from build123d import *

# Parameters (mm, degrees)
SKETCH3_R               = 25.75
SKETCH3_R_2             = 23.75
BOSS_EXTRUDE1_DEPTH     = 82
SKETCH2_R               = 24.35
SKETCH2_R_2             = 22.35
BOSS_EXTRUDE2_DEPTH     = 30
CUT_EXTRUDE1_DEPTH      = 30
CUT_EXTRUDE1_DEPTH_BACK = 30
SKETCH5_W               = 101.816386604
SKETCH5_H               = 90.816460778
CUT_EXTRUDE2_DEPTH      = 30
SKETCH6_W               = 2
SKETCH6_H               = 20.775230247
BOSS_EXTRUDE3_DEPTH     = 61
BOSS_EXTRUDE5_DEPTH     = 25


with BuildPart() as part:
    # Sketch3 → Boss-Extrude1 (new body)
    with BuildSketch(Plane(origin=(-103.870896529, 742.017814767, 0), x_dir=(-0.9903438719336157, -0.13863266326351154, 0), z_dir=(0.13863266326351156, -0.9903438719336158, 0))):
        with Locations(Location((-535.354479902, 0, 0), (0, 0, 180))):
            Circle(SKETCH3_R)
        with Locations(Location((-535.354479902, 0, 0), (0, 0, 180))):
            Circle(SKETCH3_R_2, mode=Mode.SUBTRACT)
    extrude(amount=-BOSS_EXTRUDE1_DEPTH)

    # Sketch4 → Cut-Extrude1 (cut, two sides: drawn at the far end of the back side and taken through both)
    with BuildSketch(Plane.XY.offset(-CUT_EXTRUDE1_DEPTH_BACK)):
        Polygon((414.924769966, 897.597101018), (426.314131953, 816.235432106), (451.815486656, 819.805223185), (440.426124669, 901.166892097), align=None)
    extrude(amount=CUT_EXTRUDE1_DEPTH + CUT_EXTRUDE1_DEPTH_BACK, mode=Mode.SUBTRACT)


with BuildPart() as body_2:
    # Sketch2 → Boss-Extrude2 (new body)
    with BuildSketch(Plane(origin=(455.481917253, 0, 0), x_dir=(0, 0, -1), z_dir=(1, 0, 0))):
        with Locations((0, 857.898759871)):
            Circle(SKETCH2_R)
        with Locations((0, 857.898759871)):
            Circle(SKETCH2_R_2, mode=Mode.SUBTRACT)
    extrude(amount=BOSS_EXTRUDE2_DEPTH)


with BuildPart() as cut_extrude2_tool:
    # Sketch5 → Cut-Extrude2 (new body)
    with BuildSketch(Plane.XY):
        with Locations((437.415428166, 854.729783017)):
            Rectangle(SKETCH5_W, SKETCH5_H)
    extrude(amount=-CUT_EXTRUDE2_DEPTH)


with BuildPart() as part_1:
    add(part.part)

    # Cut-Extrude2: cut by cut_extrude2_tool
    add(cut_extrude2_tool.part, mode=Mode.SUBTRACT)



with BuildPart() as body_2_1:
    add(body_2.part)

    # Cut-Extrude2: cut by cut_extrude2_tool
    add(cut_extrude2_tool.part, mode=Mode.SUBTRACT)


with BuildPart() as part_2:
    add(part_1.part)

    add(body_2_1.part)  # Boss-Extrude3 merges body 2
    # Sketch6 → Boss-Extrude3 (add)
    with BuildSketch(Plane(origin=(530.185028483, 74.217617339, 0), x_dir=(0, 0, -1), z_dir=(0.9903438719336157, 0.13863266326351165, 0))):
        with Locations((-24.75, 784.889811472)):
            Rectangle(SKETCH6_W, SKETCH6_H)
    extrude(amount=BOSS_EXTRUDE3_DEPTH)

    # Sketch7 → Boss-Extrude5 (add)
    with BuildSketch(Plane(origin=(590.596004671, 82.674209798, 0), x_dir=(0, 0, -1), z_dir=(0.9903438719336163, 0.1386326632635082, 0))):
        with BuildLine():
            Line((-23.107264421, 774.705646561), (-23.75, 774.502196348))
            Line((-23.75, 774.502196348), (-25.75, 774.502196348))
            Line((-25.75, 774.502196348), (-25.75, 795.277426595))
            Line((-25.75, 795.277426595), (-20.530540655, 795.277426595))
            ThreePointArc((-20.530540655, 795.277426595), (-24.164463247, 785.285330407), (-23.107264421, 774.705646561))
        make_face()
    extrude(amount=-BOSS_EXTRUDE5_DEPTH)


solid = part_2.part
Check sheet for the modelled part. Datum: model origin and axes. Units: mm. A direction names the side the tool comes from. Round coordinates to 2 decimals unless told otherwise and drop trailing zeros. Loops run counter-clockwise (first coordinate to the right, second up) from the corner with the lowest first, then second, coordinate; pieces in that order, holes last. Notation, with made-up numbers: (30, 79) - (57, 79) arc R33 cw to (57, 118) - close; hole circle Ø7 at (12.25, 41). An arc over 180 degrees is marked (long way). Answer as CSV lines item,"result". Start each with the question number.
Item 1: Scan lines: line 1 (Z direction, x = 433.5, y = 853.5); line 2 (Y direction, x = 459, z = 3.5); line 3 (Y direction, x = 458, z = 4.25) (3 decimals). Record each from-to range of solid material in increasing order. Write a range as [from, to].
Item 2: Section check B-B (z = 8). Record the boundary of the cut face in (x, y), and give its area (3 significant figures).
Item 3: Release check for a two-part mould opening along X. For faces 1 (the flat face through (438, 854, 23.75)), 2 (the flat face through (481.444, 862.415, 24.389)), 3 (the flat face through (470, 835, 0)) record: +X half, -X half, draft (parallel to the pull), parting line (faces both ways), or undercut.
Item 4: Section check A-A (z = 12.75). Record the boundary of the cut face in (x, y), and give its area (3 significant figures).
Item 5: Set-up check for faces 4 (the flat face through (417.405, 879.879, 24.736)), 5 (the cylindrical face through (470.272, 858.39, 22.345)), 6 (the flat face through (424.54, 828.91, 24.74)), 7 (the cylindrical face through (404.262, 853.969, 16.977)), 8 (the flat face through (471, 848.1, 23.4)): record each of +Z, -Z, +X, -X, +Y, -Y from which the full face is reachable in a straight line by a thin tool's end or side.
Item 6: Depth check by flat-ended pin: P1, Ø10, axis at x = 419, y = 870, coming from the -Z side; P2, Ø12, axis at x = 463.5, y = 838, coming from the -Z side; P3, Ø5, axis at x = 420, y = 865.5, coming from the -Z side; P4, Ø7.5, axis at x = 445, y = 854, coming from the -Z side. Enter the tip coordinate at first touch or a pass-through.
Report:
1,line 1,"z = [23.75, 25.75]"
1,line 2,"y = [833.8, 835.82], [879.97, 882]"
1,line 3,"y = [833.923, 835.957], [879.841, 881.875]"
2,outline,"(390.71, 894.05) - (402.07, 812.84) - (404.17, 813.14) - (392.8, 894.34) - close; (455.48, 834.9) - (485.48, 834.9) - (485.48, 837.03) - (455.48, 837.03) - close; (455.48, 878.77) - (485.48, 878.77) - (485.48, 880.9) - (455.48, 880.9) - close"
2,area,"301 mm2"
3,face 1,"undercut"
3,face 2,"+X half"
3,face 3,"draft"
4,outline,"(392.79, 894.34) - (404.16, 813.13) - (406.47, 813.46) - (395.1, 894.67) - close; (455.48, 837.15) - (485.48, 837.15) - (485.48, 839.54) - (455.48, 839.54) - close; (455.48, 876.26) - (485.48, 876.26) - (485.48, 878.64) - (455.48, 878.64) - close"
4,area,"335 mm2"
5,face 4,"+Z, -Z, +Y"
5,face 5,"-Z, +X"
5,face 6,"+Z, -Z, +X"
5,face 7,"-Z, +Y"
5,face 8,"+X, -Y"
6,P1,"stops at z = 23.26"
6,P2,"stops at z = 0"
6,P3,"stops at z = 23.67"
6,P4,"stops at z = 23.75"
